Answer from the drawing. Dimensions are ordinates in mm from the lowest x, y and z of the part. Give positions to 0.01 mm unless a question says otherwise; leave off trailing zeros. Order: outer loops, then holes, each group sorted by start corner. A loop starts at its lowest first (then second) coordinate and runs counter-clockwise, first axis right, second up. Notation, with made-up numbers: (40.5, -9.75) - (99.5, -9.75) arc R6 cw to (99.5, 0.25) - close; hole circle Ø1 at (-5.5, 37). An arc over 180 degrees is marked (long way). Answer in a Markdown table with one row per item.
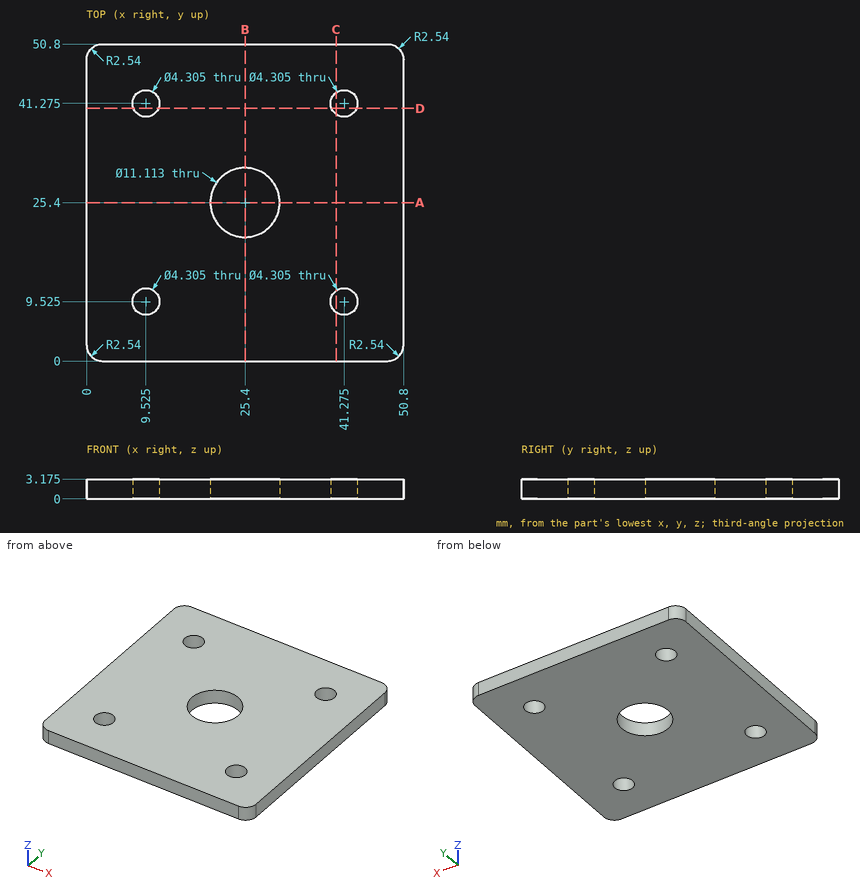
Item 1: Find section C-C on x = 40. Write down the section's boundary in (y, z) (1 decimal), then the cut area to 3 significant figures.
Answer block:
| item | result |
|---|---|
| outline | (0, 0) - (7.8, 0) - (7.8, 3.2) - (0, 3.2) - close; (11.3, 0) - (39.5, 0) - (39.5, 3.2) - (11.3, 3.2) - close; (43, 0) - (50.8, 0) - (50.8, 3.2) - (43, 3.2) - close |
| area | 139 mm² |
Item 2: Consider line 1 (Y direction, x = 9.5, z = 1.45); line 2 (Y direction, x = 25.4, z = 2); line 3 (X direction, y = 9, z = 1.65). Determine where each line is inside the solid, lowest interval first.
Answer block:
| item | result |
|---|---|
| line 1 | 0 to 7.37, 11.68 to 39.12, 43.43 to 50.8 |
| line 2 | 0 to 19.84, 30.96 to 50.8 |
| line 3 | 0 to 7.44, 11.61 to 39.19, 43.36 to 50.8 |
Item 3: Find section A-A on y = 25.4. Write down the section's boundary in (x, z) (1 decimal).
Answer block:
| item | result |
|---|---|
| outline | (0, 0) - (19.8, 0) - (19.8, 3.2) - (0, 3.2) - close; (31, 0) - (50.8, 0) - (50.8, 3.2) - (31, 3.2) - close |
Item 4: Find section D-D on y = 40.5. Write down the section's boundary in (x, z) (1 decimal).
Answer block:
| item | result |
|---|---|
| outline | (0, 0) - (7.5, 0) - (7.5, 3.2) - (0, 3.2) - close; (11.5, 0) - (39.3, 0) - (39.3, 3.2) - (11.5, 3.2) - close; (43.3, 0) - (50.8, 0) - (50.8, 3.2) - (43.3, 3.2) - close |
